Can you work these out from the model? Positions are in its coordinate system, mm. Face numbers are marked on the shaded views. A direction names the side the tool comes from. Coordinates: 2 decimals unless noted, no trailing zeros. Order: outer loops, then holes, each group sorted by start corner. A loop starts at its lowest first (then second) coordinate and runs counter-clockwise, first axis right, second up. Notation, with made-up numbers: (-16.75, 89.5) - (27.25, 89.5) arc R31 cw to (27.25, 125.5) - close; hole circle Ø5 at (80.5, 34.25). An arc over 180 degrees is marked (long way). Return JSON: item names as keys, results as strings. Group by question number.
1) Imagine slicing it at A-A (z = 24.5). Write out the boundary of the cut face in (x, y), and give its area (3 significant figures).
2) Imagine slicing it at B-B (x = -34.5). Write out the boundary of the cut face in (y, z), and give its area (3 significant figures).
3) Which directions (+Z, -Z, +X, -X, +Y, -Y) give clear straight access to the entire face, cutting with the end or side of a thin tool? Please do the marked faces 1 and 2.
4) Imagine slicing it at C-C (y = 6.75). Write out the boundary of the cut face in (x, z).
5) Imagine slicing it at D-D (z = -20.5). Write out the boundary of the cut face in (x, y).
6) If I drill on line 1 along X through (y, z) = (2.4, 24.5); line 2 along X through (y, z) = (6.75, 16.5); line 3 along Y through (x, z) = (-28, -20.5), over which ranges is the centre line in solid material (lowest first)?
7) If we mould it in two halves opening along Y, with no side actions, what happens to the marked faces 3, 4 and 5? For each: pulls with the +Y half, pulls with the -Y half, needs draft (parallel to the pull), parting line crosses it, or undercut.
8) For pin 1 Ø1.5 at (y, z) = (4, 11) entering from -X; pin 2 Ø9.5 at (x, z) = (-33.5, 3.5) entering from +Y, each with a flat end and sliding along its axis, tell me the tip position at first contact or that it passes through.
```python
from build123d import *

# Parameters (mm, degrees)
SKETCH1_W           = 77
SKETCH1_H           = 57
SKETCH1_R           = 1.5
BOSS_EXTRUDE1_DEPTH = 3
SKETCH2_W           = 65
SKETCH2_H           = 57
BOSS_EXTRUDE2_DEPTH = 20


with BuildPart() as part:
    # Sketch1 → Boss-Extrude1 (new body)
    with BuildSketch(Plane(origin=(0, 0, 0), x_dir=(1, 0, 0), z_dir=(0, 1, 0))):
        Rectangle(SKETCH1_W, SKETCH1_H)
        with Locations(Location((-34.5, 24.5, 0), (0, 0, 270))):
            Circle(SKETCH1_R, mode=Mode.SUBTRACT)
        with Locations(Location((-34.5, -24.5, 0), (0, 0, 270))):
            Circle(SKETCH1_R, mode=Mode.SUBTRACT)
    extrude(amount=BOSS_EXTRUDE1_DEPTH)

    # Sketch2 → Boss-Extrude2 (add)
    with BuildSketch(Plane(origin=(0, 3, 0), x_dir=(1, 0, 0), z_dir=(0, 1, 0))):
        with Locations((6, 0)):
            Rectangle(SKETCH2_W, SKETCH2_H)
    extrude(amount=BOSS_EXTRUDE2_DEPTH)


solid = part.part
```
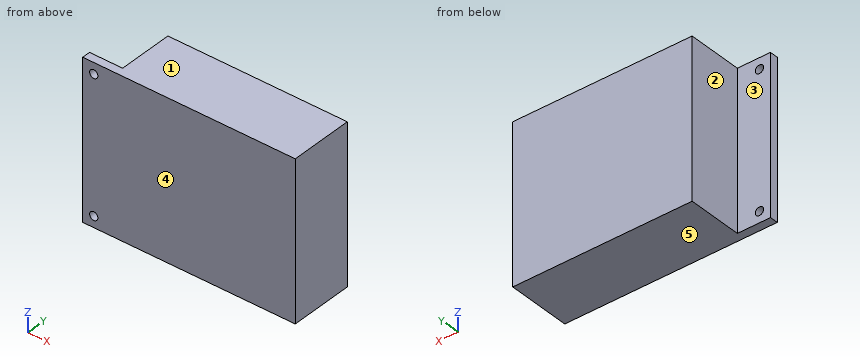
Calculated:
{
 "1": {"outline": "(-38.5, 0) - (-36, 0) - (-36, 3) - (-38.5, 3) - close; (-33, 0) - (38.5, 0) - (38.5, 23) - (-26.5, 23) - (-26.5, 3) - (-33, 3) - close", "area": "1,520 mm2"},
 "2": {"outline": "(0, -28.5) - (3, -28.5) - (3, -26) - (0, -26) - close; (0, -23) - (3, -23) - (3, 23) - (0, 23) - close; (0, 26) - (3, 26) - (3, 28.5) - (0, 28.5) - close", "area": "153 mm2"},
 "3": {"face 1": "+Z, +X, -X, +Y, -Y", "face 2": "+Z, -Z, -X, +Y"},
 "4": {"outline": "(-26.5, -28.5) - (38.5, -28.5) - (38.5, 28.5) - (-26.5, 28.5) - close"},
 "5": {"outline": "(-38.5, 0) - (38.5, 0) - (38.5, 23) - (-26.5, 23) - (-26.5, 3) - (-38.5, 3) - close"},
 "6": {"line 1": "-38.5 to -36, -33 to 38.5", "line 2": "-26.5 to 38.5", "line 3": "0 to 3"},
 "7": {"face 3": "pulls with the +Y half", "face 4": "pulls with the -Y half", "face 5": "needs draft"},
 "8": {"pin 1": "x = -26.5", "pin 2": "y = 3"}
}
